Geometry: final body of the model. Coordinates: model frame, mm. Face numbers are marked on the shaded views. A direction names the side the tool comes from. Give positions to 0.01 mm unless a question says otherwise; leave off trailing zeros. Write each loop counter-clockwise with the first axis right and the second up, starting at its lowest first coordinate (ties: lowest second). Pieces come first, ordered by that corner, then holes.
```python
from build123d import *

# Parameters (mm, degrees)
F1_DEPTH = 20
F2_R     = 5.5
F3_DEPTH = 3.5
F3_TAPER = 45
F4_R     = 2.6
F5_DEPTH = 2


with BuildPart() as f1:
    # F0 (on Top) → F1 (new body)
    with BuildSketch(Plane.XY):
        with BuildLine():
            Line((21.7278633238, -44.76), (25.7278633238, -37.8317967697))
            Line((25.7278633238, -37.8317967697), (18.9543606319, -37.5638475773))
            Line((18.9543606319, -37.5638475773), (15.9543606319, -42.76))
            ThreePointArc((15.9543606319, -42.76), (13.7582082092, -44.9561524227), (10.7582082092, -45.76))
            Line((10.7582082092, -45.76), (10, -45.76))
            Line((10, -45.76), (-10, -45.76))
            Line((-10, -45.76), (-10.7582082092, -45.76))
            ThreePointArc((-10.7582082092, -45.76), (-13.7582082092, -44.9561524227), (-15.9543606319, -42.76))
            Line((-15.9543606319, -42.76), (-18.9543606319, -37.5638475773))
            Line((-18.9543606319, -37.5638475773), (-25.7278633238, -37.8317967697))
            Line((-25.7278633238, -37.8317967697), (-21.7278633238, -44.76))
            ThreePointArc((-21.7278633238, -44.76), (-18.0676092859, -48.4202540378), (-13.0676092859, -49.76))
            Line((-13.0676092859, -49.76), (13.0676092859, -49.76))
            ThreePointArc((13.0676092859, -49.76), (18.0676092859, -48.4202540378), (21.7278633238, -44.76))
        make_face()
    extrude(amount=F1_DEPTH)

    # F2 (on face) → F3 (cut)
    with BuildSketch(Plane.XZ.offset(49.76)):
        with Locations((0, 10)):
            Circle(F2_R)
    extrude(amount=-F3_DEPTH, taper=F3_TAPER, mode=Mode.SUBTRACT)

    # F4 (on face) → F5 (cut)
    with BuildSketch(Plane(origin=(0, -45.76, 0), x_dir=(-1, 0, 0), z_dir=(0, 1, 0))):
        with Locations((0, 10)):
            Circle(F4_R)
    extrude(amount=-F5_DEPTH, mode=Mode.SUBTRACT)


solid = f1.part
```
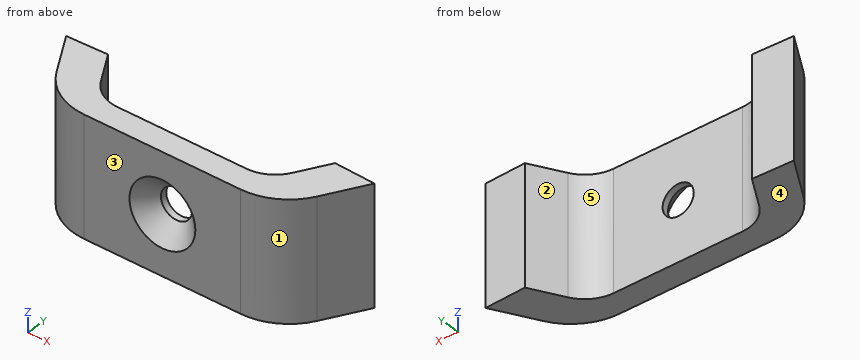
Item 1: Section C-C, the plane y = -42. Return the cut outline in (x, z), plus the area to 3 significant figures.
Found:
outline: (-23.32, 0) - (-16.39, 0) - (-16.39, 20) - (-23.32, 20) - close; (16.39, 0) - (23.32, 0) - (23.32, 20) - (16.39, 20) - close
area: 277 mm2
Item 2: Section B-B, the plane z = 17.5. Return the cut outline in (x, y), plus the area to 3 significant figures.
Found:
outline: (-25.73, -37.83) - (-21.73, -44.76) arc R10 ccw to (-13.07, -49.76) - (13.07, -49.76) arc R10 ccw to (21.73, -44.76) - (25.73, -37.83) - (18.95, -37.56) - (15.95, -42.76) arc R6 cw to (10.76, -45.76) - (-10.76, -45.76) arc R6 cw to (-15.95, -42.76) - (-18.95, -37.56) - close
area: 265 mm2
Item 3: Reachability of the marked faces 4 and 5 from +Z, -Z, +X, -X, +Y, -Y: full face, straight path, thin tool, end or side. Return the list, or none.
Found:
face 4: -Z, +X, -X, +Y, -Y
face 5: +Z, -Z, +Y
Item 4: Section D-D, the plane y = -48.25. Return the cut outline in (x, z), plus the area to 3 significant figures.
Found:
outline: (-18.35, 0) - (18.35, 0) - (18.35, 20) - (-18.35, 20) - close; hole circle Ø7.98 at (0, 10)
area: 684 mm2
Item 5: Pull-direction query (X, two-part tool) for the marked faces 1, 2 and 3; classes: +X half, -X half, draft (parallel to the pull), parting line (faces both ways), or undercut.
Found:
face 1: +X half
face 2: undercut
face 3: draft
Item 6: Line query: L1, parallel to Z at x = 0, y = -46.15; L2, parallel to X at y = -42.25, z = 10.5; L3, parallel to Y at x = -1, z = 16. Output: solid intervals per line, ascending.
Found:
L1: z = 0 to 7.4, 12.6 to 20
L2: x = -23.18 to -16.25, 16.25 to 23.18
L3: y = -49.76 to -45.76
Item 7: Pin query (flat end, axial travel): pin 1 Ø4 at (y, z) = (-41, 16) entering from +X; pin 2 Ø8.5 at (x, z) = (0, 10) entering from -Y; pin 3 Ø6 at (y, z) = (-43.5, 12) entering from -X. Return the tip coordinate at first contact, or that it passes through.
Found:
pin 1: stops at x = 25.05
pin 2: stops at y = -48.51
pin 3: stops at x = -24.19
Item 8: Section A-A, the plane x = 0. Return the cut outline in (y, z), plus the area to 3 significant figures.
Found:
outline: (-49.76, 0) - (-45.76, 0) - (-45.76, 7.4) - (-46.86, 7.4) - (-49.76, 4.5) - close; (-49.76, 15.5) - (-46.86, 12.6) - (-45.76, 12.6) - (-45.76, 20) - (-49.76, 20) - close
area: 50.8 mm2
